Autodesk Inventor part; units mm, degrees
ref_plane "YZ Plane" through (0, 0, 0) normal (1, 0, 0) x (0, 1, 0)
ref_plane "XZ Plane" through (0, 0, 0) normal (0, 1, 0) x (-1, 0, 0)
ref_plane "XY Plane" through (0, 0, 0) normal (0, 0, 1) x (1, 0, 0)
sketch "Sketch1" plane through (0, 0, 0) normal (0, 0, 1) x (1, 0, 0)
  line L0 (0, 0) -> (108, 0)
  line L1 (108, 0) -> (108, 40)
  line L2 (108, 40) -> (0, 40)
  line L3 (0, 40) -> (0, 0)
  line L4 (13.854, 37) -> (19.146, 37)
  line L5 (19.146, 37) -> (19.146, 29)
  line L6 (19.146, 29) -> (13.854, 29)
  line L7 (13.854, 29) -> (13.854, 37)
  line L8 (13.854, 11) -> (19.146, 11)
  line L9 (19.146, 11) -> (19.146, 3)
  line L10 (19.146, 3) -> (13.854, 3)
  line L11 (13.854, 3) -> (13.854, 11)
  line L12 (88.854, 37) -> (94.146, 37)
  line L13 (94.146, 37) -> (94.146, 29)
  line L14 (94.146, 29) -> (88.854, 29)
  line L15 (88.854, 29) -> (88.854, 37)
  line L16 (88.854, 11) -> (94.146, 11)
  line L17 (94.146, 11) -> (94.146, 3)
  line L18 (94.146, 3) -> (88.854, 3)
  line L19 (88.854, 3) -> (88.854, 11)
  dimension "d0" = 40
  dimension "d1" = 108
  dimension "d73" = 8
  dimension "d74" = 5.292
  dimension "d75" = 3
  dimension "d76" = 13.854
  dimension "d77" = 5.292
  dimension "d78" = 8
  dimension "d79" = 3
  dimension "d80" = 5.292
  dimension "d81" = 8
  dimension "d82" = 13.854
  dimension "d83" = 3
  dimension "d84" = 5.292
  dimension "d85" = 13.854
extrude "Extrusion1" add sketch "Sketch1" along normal blind 3
sketch "Sketch3" plane through (0, 0, 3) normal (0, 0, 1) x (1, 0, 0)
  line L0 (0, 0) -> (0, 40)
  line L1 (108, 0) -> (0, 0)
  line L2 (0, 40) -> (108, 40)
  point P0 (54, 26.5)
  point P1 (54, 13.5)
  dimension "d56" = 54
  dimension "d57" = 13.5
  dimension "d58" = 13.5
  dimension "d59" = 54
hole "Hole1" at (54, 26.5, 3) at (54, 13.5, 3) direction (0, 0, -1) diameter 3 end through all
sketch "Sketch8" plane through (0, 0, 3) normal (0, 0, 1) x (1, 0, 0)
  line L0 (108, 0) -> (0, 0)
  line L1 (0, 40) -> (108, 40)
  line L2 (28, 40) -> (80, 40)
  line L3 (80, 40) -> (80, 30)
  line L4 (80, 30) -> (28, 30)
  line L5 (28, 30) -> (28, 40)
  line L6 (28, 0) -> (80, 0)
  line L7 (80, 0) -> (80, 10)
  line L8 (80, 10) -> (28, 10)
  line L9 (28, 10) -> (28, 0)
  line L10 (108, 40) -> (108, 0)
  line L11 (0, 0) -> (0, 40)
  dimension "d68" = 10
  dimension "d69" = 10
  dimension "d87" = 28
  dimension "d88" = 28
  dimension "d130" = 28
  dimension "d131" = 28
extrude "Extrusion5" cut sketch "Sketch8" against normal through all contours L0 L9 L8 L7 | L3 L4 L5 L1
fillet "Fillet3" radius 2 8 edges at (28, 40, 1.5) (28, 0, 1.5) (28, 10, 1.5) (28, 30, 1.5) (80, 10, 1.5) (80, 30, 1.5) (80, 0, 1.5) (80, 40, 1.5)
fillet "Fillet4" radius 5 4 edges at (0, 0, 1.5) (0, 40, 1.5) (108, 0, 1.5) (108, 40, 1.5)
sketch "Sketch12" plane through (0, 0, 3) normal (0, 0, 1) x (1, 0, 0)
  arc A0 (5, 40) -> (0, 35) centre (5, 35) ccw
  arc A1 (0, 5) -> (5, 0) centre (5, 5) ccw
  arc A2 (103, 0) -> (108, 5) centre (103, 5) ccw
  arc A3 (108, 35) -> (103, 40) centre (103, 35) ccw
  circle A4 centre (54, 26.5) radius 1.5
  line L0 (78, 30) -> (30, 30)
  point P0 (41.5, 20)
  dimension "d141" = 12.5
  dimension "d142" = 10
hole "Hole4" at (5, 35, 3) at (5, 5, 3) at (103, 35, 3) at (103, 5, 3) at (41.5, 20, 3) direction (0, 0, -1) diameter 3 end through all
sketch "草圖14" plane through (0, 0, 3) normal (0, 0, 1) x (1, 0, 0)
  line L0 (94.146, 37) -> (94.146, 29)
  line L1 (88.854, 29) -> (88.854, 37)
  line L2 (19.146, 37) -> (19.146, 29)
  line L3 (13.854, 29) -> (13.854, 37)
  line L4 (13.854, 37) -> (19.146, 37)
  line L5 (13.854, 11) -> (19.146, 11)
  line L6 (9.8, 34.25) -> (11.2, 34.25)
  line L7 (11.2, 34.25) -> (11.2, 31.75)
  line L8 (11.2, 31.75) -> (9.8, 31.75)
  line L9 (9.8, 31.75) -> (9.8, 34.25)
  line L10 (21.8, 34.25) -> (23.2, 34.25)
  line L11 (23.2, 34.25) -> (23.2, 31.75)
  line L12 (23.2, 31.75) -> (21.8, 31.75)
  line L13 (21.8, 31.75) -> (21.8, 34.25)
  line L14 (9.8, 8.25) -> (11.2, 8.25)
  line L15 (11.2, 8.25) -> (11.2, 5.75)
  line L16 (11.2, 5.75) -> (9.8, 5.75)
  line L17 (9.8, 5.75) -> (9.8, 8.25)
  line L18 (21.8, 8.25) -> (23.2, 8.25)
  line L19 (23.2, 8.25) -> (23.2, 5.75)
  line L20 (23.2, 5.75) -> (21.8, 5.75)
  line L21 (21.8, 5.75) -> (21.8, 8.25)
  line L22 (84.8, 34.25) -> (86.2, 34.25)
  line L23 (86.2, 34.25) -> (86.2, 31.75)
  line L24 (86.2, 31.75) -> (84.8, 31.75)
  line L25 (84.8, 31.75) -> (84.8, 34.25)
  line L26 (96.8, 34.25) -> (98.2, 34.25)
  line L27 (98.2, 34.25) -> (98.2, 31.75)
  line L28 (98.2, 31.75) -> (96.8, 31.75)
  line L29 (96.8, 31.75) -> (96.8, 34.25)
  line L30 (84.8, 8.25) -> (86.2, 8.25)
  line L31 (86.2, 8.25) -> (86.2, 5.75)
  line L32 (86.2, 5.75) -> (84.8, 5.75)
  line L33 (84.8, 5.75) -> (84.8, 8.25)
  line L34 (96.8, 8.25) -> (98.2, 8.25)
  line L35 (98.2, 8.25) -> (98.2, 5.75)
  line L36 (98.2, 5.75) -> (96.8, 5.75)
  line L37 (96.8, 5.75) -> (96.8, 8.25)
  point P0 (0, 0)
  dimension "d143" = 1.4
  dimension "d145" = 2.654
  dimension "d146" = 2.75
  dimension "d147" = 2.5
  dimension "d148" = 1.4
  dimension "d149" = 2.654
  dimension "d150" = 2.5
  dimension "d151" = 1.4
  dimension "d152" = 2.75
  dimension "d153" = 1.4
  dimension "d154" = 2.5
  dimension "d155" = 2.654
  dimension "d156" = 2.654
  dimension "d157" = 1.4
  dimension "d158" = 1.4
  dimension "d159" = 1.4
extrude "擠出7" cut sketch "草圖14" against normal through all
properties part number "plastic_part_12"
Here's how the part is built. I have some questions about the finished solid (model axes, mm). A direction names the side the tool comes from. Coordinates: 2 decimals unless noted, no trailing zeros. Loops run counter-clockwise (first coordinate to the right, second up) from the corner with the lowest first, then second, coordinate; pieces in that order, holes last. Notation, with made-up numbers: (58, -25) -> (71, -25) arc R17 ccw to (71, 1) -> close; hole circle Ø11 at (-4, 76). An arc over 180 degrees is marked (long way). Return JSON: item names as keys, results as strings.
1) If we section it at D-D, the plane y = 20.5: Write out the boundary of the cut face in (x, z), then the cut area to 3 significant figures.
Results below:
{"outline": "(0, 0) -> (40.09, 0) -> (40.09, 3) -> (0, 3) -> close; (42.91, 0) -> (108, 0) -> (108, 3) -> (42.91, 3) -> close", "area": "316 mm²"}
2) Will this pin go through, and if not, where does the flat tip stop? pin 1 (1 mm diameter, centred on x = 43.5, y = 32, fed in from -Z).
Results below:
{"pin 1": "through"}
3) If we section it at B-B, the plane y = 13.5: Write out the boundary of the cut face in (x, z).
Results below:
{"outline": "(0, 0) -> (52.5, 0) -> (52.5, 3) -> (0, 3) -> close; (55.5, 0) -> (108, 0) -> (108, 3) -> (55.5, 3) -> close"}
4) For faces 1 (the face through (88.854, 33, 1)), 2 (the face through (28.6, 30.57, 1.48)), 3 (the face through (53, 20, 3)), which set-ups out of +Z, -Z, +X, -X, +Y, -Y let a thin tool reach every point of the face, with its end or its side?
Results below:
{"face 1": "+Z, -Z", "face 2": "+Z, -Z, +Y", "face 3": "+Z, +X, -X, +Y, -Y"}
5) I need wall thicknesses on line 1 (X direction, y = 35, z = 2.35); line 2 (Y direction, x = 103, z = 0.7); line 3 (Y direction, x = 90, z = 2.35). Which ranges of each line are inside material? Lowest first, please. Write a range as from..to.
Results below:
{"line 1": "0..3.5, 6.5..13.85, 19.15..28, 80..88.85, 94.15..101.5, 104.5..108", "line 2": "0..3.5, 6.5..33.5, 36.5..40", "line 3": "0..3, 11..29, 37..40"}
6) If we section it at A-A, the plane x = 54: Write out the boundary of the cut face in (y, z), then the cut area to 3 significant figures.
Results below:
{"outline": "(10, 0) -> (12, 0) -> (12, 3) -> (10, 3) -> close; (15, 0) -> (25, 0) -> (25, 3) -> (15, 3) -> close; (28, 0) -> (30, 0) -> (30, 3) -> (28, 3) -> close", "area": "42.0 mm²"}
7) Thinking about a two-plate mould opening in Y: for faces 4 (the face through (108, 20, 1)), 5 (the face through (11.2, 7, 2)), 6 (the face through (79.4, 9.43, 1.48)), which applies, +Y half, -Y half, draft (parallel to the pull), parting line (faces both ways), or undercut?
Results below:
{"face 4": "draft", "face 5": "undercut", "face 6": "-Y half"}
8) If we section it at C-C, the plane z = 2: Count the separate pieces of the cut face and the enclosed holes in it, then the cut area to 3 significant figures.
Results below:
{"separate pieces": "1", "enclosed holes": "19", "area": "3,010 mm²"}
